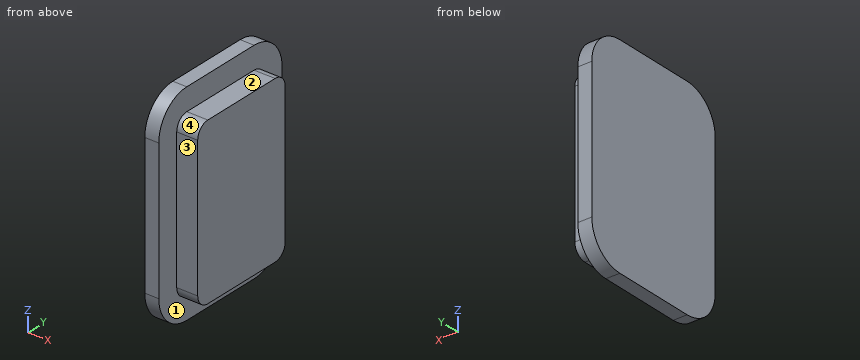
from build123d import *

# Parameters (mm, degrees)
BOSS_EXTRUDE1_DEPTH = 1
BOSS_EXTRUDE2_DEPTH = 1.5


with BuildPart() as part:
    # Sketch1 → Boss-Extrude1 (new body)
    with BuildSketch(Plane.ZY.offset(60)):
        with BuildLine():
            Line((-36.32233047, 7.85), (-26.32233047, 7.85))
            ThreePointArc((-26.32233047, 7.85), (-24.554563517, 8.582233047), (-23.82233047, 10.35))
            Line((-23.82233047, 10.35), (-23.82233047, 16.35))
            ThreePointArc((-23.82233047, 16.35), (-24.554563517, 18.117766953), (-26.32233047, 18.85))
            Line((-26.32233047, 18.85), (-36.32233047, 18.85))
            ThreePointArc((-36.32233047, 18.85), (-38.090097423, 18.117766953), (-38.82233047, 16.35))
            Line((-38.82233047, 16.35), (-38.82233047, 10.35))
            ThreePointArc((-38.82233047, 10.35), (-38.090097423, 8.582233047), (-36.32233047, 7.85))
        make_face()
    extrude(amount=BOSS_EXTRUDE1_DEPTH)

    # Sketch1<3> → Boss-Extrude2 (add)
    with BuildSketch(Plane.ZY.offset(60)):
        with BuildLine():
            Line((-36.32233047, 9.45), (-26.32233047, 9.45))
            ThreePointArc((-26.32233047, 9.45), (-25.685934367, 9.713603897), (-25.42233047, 10.35))
            Line((-25.42233047, 10.35), (-25.42233047, 16.35))
            ThreePointArc((-25.42233047, 16.35), (-25.685934367, 16.986396103), (-26.32233047, 17.25))
            Line((-26.32233047, 17.25), (-36.32233047, 17.25))
            ThreePointArc((-36.32233047, 17.25), (-36.958726573, 16.986396103), (-37.22233047, 16.35))
            Line((-37.22233047, 16.35), (-37.22233047, 10.35))
            ThreePointArc((-37.22233047, 10.35), (-36.958726573, 9.713603897), (-36.32233047, 9.45))
        make_face()
    extrude(amount=-BOSS_EXTRUDE2_DEPTH)


solid = part.part
Read the model definition and answer for the solid it produces. Units are mm, in the model's axes. Face numbers are marked on the shaded views. A direction names the side the tool comes from. Round coordinates to 2 decimals unless told otherwise and drop trailing zeros. Write each loop counter-clockwise with the first axis right and the second up, starting at its lowest first coordinate (ties: lowest second). Pieces come first, ordered by that corner, then holes.
1. Given pin 1 Ø0.8 at (x, z) = (-59, -29) entering from +Y; pin 2 Ø0.8 at (x, y) = (-59, 12) entering from -Z, each flat-ended and moving along its own axis, determine where each tip first touches the part or whether it passes through.
2. The part is cut by section B-B, the plane y = 16. Determine the outline of the cut face in (x, z).
3. The part is cut by section C-C, the plane y = 9.25. Determine the outline of the cut face in (x, z).
4. The part is cut by section A-A, the plane x = -59.25. Determine the outline of the cut face in (y, z).
5. Straight lines are drawn through the part: L1, parallel to X at y = 18, z = -36.75; L2, parallel to Z at x = -59.15, y = 13.5; L3, parallel to Y at x = -59.8, z = -34.75. For each, find the intervals that lie inside material, in ascending order.
6. Which of the six approach directions +Z, -Z, +X, -X, +Y, -Y give full straight-line access (tool end or side, diameter ignored) to the marked faces 1, 2, 3 and 4?
7. The part is cut by section D-D, the plane y = 18. Determine the outline of the cut face in (x, z).
Values:
1. pin 1: stops at y = 17.25
1. pin 2: stops at z = -37.22
2. outline: (-61, -38.82) - (-60, -38.82) - (-60, -37.22) - (-58.5, -37.22) - (-58.5, -25.42) - (-60, -25.42) - (-60, -23.82) - (-61, -23.82) - close
3. outline: (-61, -38.57) - (-60, -38.57) - (-60, -24.08) - (-61, -24.08) - close
4. outline: (9.45, -36.32) arc R0.9 ccw to (10.35, -37.22) - (16.35, -37.22) arc R0.9 ccw to (17.25, -36.32) - (17.25, -26.32) arc R0.9 ccw to (16.35, -25.42) - (10.35, -25.42) arc R0.9 ccw to (9.45, -26.32) - close
5. L1: x = -61 to -60
5. L2: z = -37.22 to -25.42
5. L3: y = 9.45 to 17.25
6. face 1: +X
6. face 2: +Z, +X, +Y, -Y
6. face 3: +Z, -Z, +X, -Y
6. face 4: +Z, +X, -Y
7. outline: (-61, -38.2) - (-60, -38.2) - (-60, -24.44) - (-61, -24.44) - close
